from build123d import *

# Parameters (mm, degrees)
F0_W     = 135.774552
F0_H     = 93.844176
F0_W_2   = 120.37155
F0_H_2   = 81.29359
F1_DEPTH = 76.2
F2_R     = 13.454778
F3_DEPTH = 135.775553
F4_W     = 74.733056
F4_H     = 47.146207
F5_DEPTH = 93.845175


with BuildPart() as f1:
    # F0 (on Top) → F1 (new body)
    with BuildSketch(Plane.XY):
        Rectangle(F0_W, F0_H)
        Rectangle(F0_W_2, F0_H_2, mode=Mode.SUBTRACT)
    extrude(amount=F1_DEPTH)

    # F2 (on face) → F3 (cut, through all)
    with BuildSketch(Plane.YZ.offset(67.887276)):
        with Locations((0, 40.932029)):
            Circle(F2_R)
    extrude(amount=-F3_DEPTH, mode=Mode.SUBTRACT)

    # F4 (on face) → F5 (cut, through all)
    with BuildSketch(Plane.XZ.offset(46.922088)):
        with Locations((0, 52.626897)):
            Rectangle(F4_W, F4_H)
    extrude(amount=-F5_DEPTH, mode=Mode.SUBTRACT)


solid = f1.part
Verification items for the finished model (mm, model axes). A direction names the side the tool comes from. Coordinates: 2 decimals unless noted, no trailing zeros. Order: outer loops, then holes, each group sorted by start corner. A loop starts at its lowest first (then second) coordinate and runs counter-clockwise, first axis right, second up. Notation, with made-up numbers: M 49,44.25 L 78,44.25 A37 cw 78,81.25 Z; hole C 26,60.25 d6. An arc over 180 degrees is marked long. Return JSON: item names as keys, results as strings.
1) Cross-section at C-C, the plane z = 12. Record the boundary of the cut face in (x, y).
Answer list:
{"outline": "M -67.89,-46.92 L 67.89,-46.92 L 67.89,46.92 L -67.89,46.92 Z; hole M -60.19,-40.65 L 60.19,-40.65 L 60.19,40.65 L -60.19,40.65 Z"}
2) Thickness scan on L1, parallel to Y at x = -3.5, z = 16; L2, parallel to X at y = -4, z = 8.5; L3, parallel to Z at x = 65, y = 0. Record the ranges inside material, lowest first. Write a range as [from, to].
Answer list:
{"L1": "[-46.92, -40.65], [40.65, 46.92]", "L2": "[-67.89, -60.19], [60.19, 67.89]", "L3": "[0, 27.48], [54.39, 76.2]"}
3) Cross-section at B-B, the plane y = 0. Record the boundary of the cut face in (x, z).
Answer list:
{"outline": "M -67.89,0 L -60.19,0 L -60.19,27.48 L -67.89,27.48 Z; M -67.89,54.39 L -60.19,54.39 L -60.19,76.2 L -67.89,76.2 Z; M 60.19,0 L 67.89,0 L 67.89,27.48 L 60.19,27.48 Z; M 60.19,54.39 L 67.89,54.39 L 67.89,76.2 L 60.19,76.2 Z"}
4) Access from +Z, -Z, +X, -X, +Y, -Y to the whole of each face (thin tool, end or side, straight path). Record for faces 1 (the flat face through (60.186, -10, 29)), 2 (the flat face through (-1, -44, 29.054)), 3 (the flat face through (-15, -41, 0)).
Answer list:
{"face 1": "+Z, -Z", "face 2": "+Z, +Y, -Y", "face 3": "-Z, +X, -X, +Y, -Y"}
5) Gauge pin test, flat ends, axial feed: pin 1 (5 mm diameter, centred on x = -11, y = -44, fed in from +Z); pin 2 (10 mm diameter, centred on x = 13, y = 35, fed in from -Z). Record the tip position at first contact, or that the pin passes through.
Answer list:
{"pin 1": "z = 29.05", "pin 2": "through"}
6) Cross-section at D-D, the plane x = 44.5. Record the boundary of the cut face in (y, z), and give its area (3 significant figures).
Answer list:
{"outline": "M -46.92,0 L -40.65,0 L -40.65,76.2 L -46.92,76.2 Z; M 40.65,0 L 46.92,0 L 46.92,76.2 L 40.65,76.2 Z", "area": "956 mm2"}
7) Cross-section at A-A, the plane x = -6. Record the boundary of the cut face in (y, z), and give its area (3 significant figures).
Answer list:
{"outline": "M -46.92,0 L -40.65,0 L -40.65,29.05 L -46.92,29.05 Z; M 40.65,0 L 46.92,0 L 46.92,29.05 L 40.65,29.05 Z", "area": "365 mm2"}
8) Release check for a two-part mould opening along Y. For faces 4 (the flat face through (-1, 40.647, 21)), 5 (the flat face through (37.367, -44, 52)), 6 (the flat face through (-1, 46.922, 21)), 7 (the cylindrical face through (-63.983, -2.917, 27.797)) record: +Y half, -Y half, draft (parallel to the pull), parting line (faces both ways), or undercut.
Answer list:
{"face 4": "undercut", "face 5": "draft", "face 6": "+Y half", "face 7": "undercut"}
